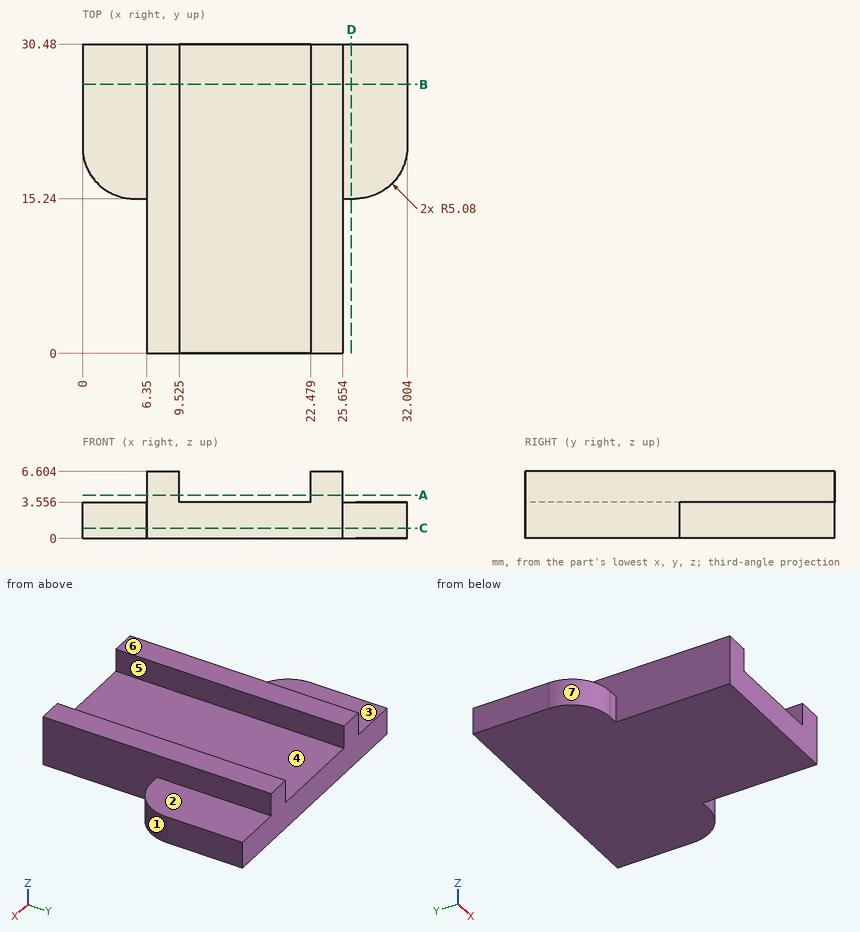
Source: three-view drawing plus pictorial views. Frame: mm from the lowest corner of the part. A direction names the side the tool comes from. Coordinates: 2 decimals unless noted, no trailing zeros. Order: outer loops, then holes, each group sorted by start corner. A loop starts at its lowest first (then second) coordinate and runs counter-clockwise, first axis right, second up.
Item 1: First-contact query: P1, Ø1, axis at x = 6, z = 1.5, coming from the -Y side; P2, Ø0.6, axis at x = 26, z = 2.5, coming from the -Y side; P3, Ø2.5, axis at y = 9, z = 5.5, coming from the +X side; P4, Ø1.9, axis at x = 2.5, y = 22.5, coming from the +Z side. Flat tips, straight axial feed; report the tip coordinate or a pass-through.
Output values:
P1: stops at y = 0
P2: stops at y = 15.24
P3: stops at x = 25.65
P4: stops at z = 3.56
Item 2: Material intervals for line 1 (X direction, y = 15.5, z = 3.75) (3 decimals); line 2 (X direction, y = 10, z = 3); line 3 (Z direction, x = 27, y = 28), sorted ascending.
Output values:
line 1: x = 6.35 to 9.525, 22.479 to 25.654
line 2: x = 6.35 to 25.65
line 3: z = 0 to 3.56
Item 3: Cut plane D-D (x = 26.5). Return loops of the section in (y, z).
Output values:
outline: (15.24, 0) - (30.48, 0) - (30.48, 3.56) - (15.24, 3.56) - close
Item 4: Cut plane A-A (z = 4.25). Return loops of the section in (x, y) (3 decimals).
Output values:
outline: (6.35, 0) - (9.525, 0) - (9.525, 30.48) - (6.35, 30.48) - close; (22.479, 0) - (25.654, 0) - (25.654, 30.48) - (22.479, 30.48) - close
Item 5: Cut plane B-B (y = 26.5). Return loops of the section in (x, z) (3 decimals), plus the area to 3 significant figures.
Output values:
outline: (0, 0) - (32.004, 0) - (32.004, 3.556) - (25.654, 3.556) - (25.654, 6.604) - (22.479, 6.604) - (22.479, 3.556) - (9.525, 3.556) - (9.525, 6.604) - (6.35, 6.604) - (6.35, 3.556) - (0, 3.556) - close
area: 133 mm2
Item 6: Pull-direction query (X, two-part tool) for the marked faces 5, 6 and 7; classes: pulls with the +X half, pulls with the -X half, needs draft (parallel to the pull), parting line crosses it, or undercut.
Output values:
face 5: undercut
face 6: needs draft
face 7: pulls with the -X half
Item 7: Set-up query: the marked faces 1, 2, 3 and 4. Return all of +Z, -Z, +X, -X, +Y, -Y with unobstructed straight access to the full face (end or side cutting, diameter ignored); none if empty.
Output values:
face 1: +Z, -Z, +X, -Y
face 2: +Z, +X, +Y, -Y
face 3: +Z, -X, +Y, -Y
face 4: +Z, +Y, -Y
Item 8: Cut plane C-C (z = 1). Return loops of the section in (x, y).
Output values:
outline: (0, 20.32) arc R5.08 ccw to (5.08, 15.24) - (6.35, 15.24) - (6.35, 0) - (25.65, 0) - (25.65, 15.24) - (26.92, 15.24) arc R5.08 ccw to (32, 20.32) - (32, 30.48) - (0, 30.48) - close
